Autodesk Inventor part; units mm, degrees
ref_plane "YZ Plane" through (0, 0, 0) normal (1, 0, 0) x (0, 1, 0)
ref_plane "XZ Plane" through (0, 0, 0) normal (0, 1, 0) x (-1, 0, 0)
ref_plane "XY Plane" through (0, 0, 0) normal (0, 0, 1) x (1, 0, 0)
sketch "Sketch1" plane through (0, 0, 0) normal (0, 0, 1) x (1, 0, 0)
  circle A0 centre (0, 0) radius 17.5
  circle A1 centre (0, -70) radius 17.5
  line L0 (-17.5, 0) -> (-17.5, -70)
  line L1 (17.5, 0) -> (17.5, -70)
  circle A2 centre (0, -70) radius 11.5 construction
  circle A3 centre (0, -70) radius 9.715 construction
  line L2 (0, -20) -> (0, -150) construction
  line L3 (11.5, -70) -> (-11.5, -70) construction
  line L4 (9.9593, -64.25) -> (0, -70) construction
  line L5 (0, -70) -> (-9.9593, -64.25) construction
  line L6 (0, -70) -> (9.9593, -75.75) construction
  line L7 (0, -70) -> (-9.9593, -75.75) construction
  circle A4 centre (0, -58.5) radius 2.75
  circle A5 centre (9.9593, -75.75) radius 2.75
  circle A6 centre (-9.9593, -75.75) radius 2.75
  circle A7 centre (0, -58.5) radius 1.65
  circle A8 centre (9.9593, -75.75) radius 1.65
  circle A9 centre (-9.9593, -75.75) radius 1.65
  circle A10 centre (8.4134, -65.1425) radius 2
  circle A11 centre (0, -79.715) radius 2
  circle A12 centre (-8.4134, -65.1425) radius 2
  line L8 (-17.5, -35) -> (17.5, -35) construction
  circle A13 centre (0, 0) radius 17.5
  line L9 (9.9593, -5.75) -> (0, 0) construction
  circle A14 centre (8.4134, -4.8575) radius 2
  line L10 (0, 0) -> (9.9593, 5.75) construction
  line L11 (0, 0) -> (-9.9593, -5.75) construction
  circle A15 centre (-8.4134, -4.8575) radius 2
  circle A16 centre (0, 0) radius 9.715 construction
  circle A17 centre (0, 0) radius 11.5 construction
  circle A18 centre (0, 9.715) radius 2
  line L12 (0, 0) -> (-9.9593, 5.75) construction
  line L13 (11.5, 0) -> (-11.5, 0) construction
  circle A19 centre (-9.9593, 5.75) radius 2.75
  circle A20 centre (-9.9593, 5.75) radius 1.65
  line L14 (0, -50) -> (0, 80) construction
  circle A21 centre (0, -11.5) radius 1.65
  circle A22 centre (0, -11.5) radius 2.75
  circle A23 centre (9.9593, 5.75) radius 2.75
  circle A24 centre (9.9593, 5.75) radius 1.65
  dimension "d3" = 23
  dimension "d0" = 35
  dimension "d1" = 70
  dimension "d2" = 19.43
  dimension "d4" = 30
  dimension "d5" = 30
  dimension "d6" = 30
  dimension "d7" = 30
  dimension "d8" = 5.5
  dimension "d9" = 3.3
  dimension "d10" = 4
extrude "Extrusion1" add sketch "Sketch1" along normal blind 12 contours A0 | L1 A1 L0 A0 | A1 | A4 | A5 | A6 | A10 | A11 | A12 | A14 | A15 | A18 | A19 | A22 | A23
extrude "Extrusion2" cut sketch "Sketch1" along normal blind 5 contours A4 | A5 | A6 | A19 | A22 | A23 | A24
extrude "Extrusion3" cut sketch "Sketch1" against normal blind 5 from surface at 12 contours A14 | A15 | A18
properties part number "shank_thigh_connector"
Model file for the job. Use its own axes, mm. A direction names the side the tool comes from. Give positions to 0.01 mm unless a question says otherwise; leave off trailing zeros. Write each loop counter-clockwise with the first axis right and the second up, starting at its lowest first coordinate (ties: lowest second). Pieces come first, ordered by that corner, then holes. Notation, with made-up numbers: M 43,24 L 83,24 A19 cw 83,53 Z; hole C 49.5,65.25 d3. An arc over 180 degrees is marked long. One line per item, written item: value. Start each with the question number.
Q1. Saw through at D-D, the plane z = 10.5. State how many separate pieces and enclosed holes the cut face has, plus the area to 3 significant figures.
Q2. Saw through at C-C, the plane z = 3. Write the cut outline in (x, y), plus the area to 3 significant figures.
Q3. 3-axis set-ups, long thin cutter, end or side, ignore diameter. For faces 5 (the cylindrical face through (-0.4, -56.9, 8.5)), 6 (the flat face through (0, 10, 7)), 7 (the flat face through (-8, -76, 5)): which of +Z, -Z, +X, -X, +Y, -Y reach the whole face in a straight line?
Q4. Saw through at A-A, the plane y = -58.5. Write the cut outline in (x, z), plus the area to 3 significant figures.
Q5. Saw through at B-B, the plane x = 0. Write the cut outline in (y, z) (3 decimals).
Q6. Probe probe 1 along Y at (x, z) = (0, 9.75) (3 decimals); probe 2 along Y at (x, z) = (11, 8); probe 3 along Y at (x, z) = (7.5, 4.25). List the from-to ranges inside material, lowest first. Write a range as [from, to].
Q7. Drop flat-ended pins along their axis: pin 1 Ø1.2 at (x, y) = (-8.5, -4.5) entering from +Z; pin 2 Ø4.5 at (x, y) = (0, -58.5) entering from -Z; pin 3 Ø3 at (x, z) = (3, 8.5) entering from +Y. Give the stop position or say it passes through.
Q8. Two-plate mould, pull along X, no slides. Class faces 1 (the cylindrical face through (-0.385, 17.496, 5.916)), 2 (the cylindrical face through (8.153, -2.875, 9.535)), 3 (the cylindrical face through (-8.435, 6.382, 8.451)), 4 (the flat face through (17.5, -35, 6)): +X half, -X half, draft (parallel to the pull), parting line (faces both ways), or undercut.
Output values:
1. separate pieces: 1
1. enclosed holes: 9
1. area: 3,320 mm²
2. outline: M -17.5,-70 A17.5 ccw 17.5,-70 L 17.5,0 A17.5 ccw -17.5,0 Z; hole C -9.96,-75.75 d5.5; hole C -9.96,5.75 d5.5; hole C 0,-58.5 d5.5; hole C 0,-11.5 d5.5; hole C 9.96,-75.75 d5.5; hole C 9.96,5.75 d5.5
2. area: 3,270 mm²
3. face 5: +Z, -Z
3. face 6: +Z
3. face 7: -Z
4. outline: M -17.5,0 L -2.75,0 L -2.75,5 L -1.65,5 L -1.65,12 L -17.5,12 Z; M 1.65,5 L 2.75,5 L 2.75,0 L 17.5,0 L 17.5,12 L 1.65,12 Z
4. area: 369 mm²
5. outline: M -87.5,0 L -61.25,0 L -61.25,5 L -60.15,5 L -60.15,12 L -87.5,12 Z; M -56.85,5 L -55.75,5 L -55.75,0 L -14.25,0 L -14.25,5 L -13.15,5 L -13.15,12 L -56.85,12 Z; M -9.85,5 L -8.75,5 L -8.75,0 L 17.5,0 L 17.5,12 L 11.715,12 L 11.715,7 L 7.715,7 L 7.715,12 L -9.85,12 Z
6. probe 1: y = [-87.5, -60.15], [-56.85, -13.15], [-9.85, 7.715], [11.715, 17.5]
6. probe 2: y = [-83.61, -77.03], [-74.47, 4.47], [7.03, 13.61]
6. probe 3: y = [-85.81, -76.98], [-74.52, 4.52], [6.98, 15.81]
7. pin 1: stops at z = 7
7. pin 2: stops at z = 5
7. pin 3: stops at y = 17.44
8. face 1: parting line
8. face 2: undercut
8. face 3: undercut
8. face 4: +X half
